Autodesk Inventor part; units mm, degrees
ref_plane "YZ Plane" through (0, 0, 0) normal (1, 0, 0) x (0, 1, 0)
ref_plane "XZ Plane" through (0, 0, 0) normal (0, 1, 0) x (-1, 0, 0)
ref_plane "XY Plane" through (0, 0, 0) normal (0, 0, 1) x (1, 0, 0)
sketch "Skizze1" plane through (0, 0, 0) normal (0, 0, 1) x (1, 0, 0)
  line L0 (-68.016, 1.808) -> (67.584, 1.808)
  line L1 (67.584, 1.808) -> (67.584, -2.192)
  line L2 (67.584, -2.192) -> (-68.016, -2.192)
  line L3 (-68.016, -2.192) -> (-68.016, 1.808)
  line L4 (-68.016, 1.808) -> (67.584, -2.192) construction
  line L5 (67.584, 1.808) -> (-68.016, -2.192) construction
  point P0 (0, 0)
  point P1 (-0.216, -0.192)
  point P2 (-0.216, -0.192)
  dimension "d0" = 135.6
  dimension "d1" = 4
extrude "Extrusion1" add sketch "Skizze1" along normal mid plane 3.25
ref_plane "Arbeitsebene1" through (-68.016, -0.192, 1.625) normal (0, -1, 0) x (1, 0, 0)
sketch "Skizze2" plane through (-68.016, -0.192, 1.625) normal (0, -1, 0) x (1, 0, 0)
  line L0 (0, -3.25) -> (0, 0)
  line L1 (0, -3.25) -> (135.6, -3.25)
  line L2 (0, 0) -> (2.85, 0)
  line L3 (2.85, 0) -> (2.85, -3.25)
  line L4 (2.85, -3.25) -> (0, -3.25)
  line L5 (0, -3.25) -> (0, 0)
  line L6 (0, 0) -> (0, 1.75)
  line L7 (0, 1.75) -> (2.85, 0)
  line L8 (135.6, -3.25) -> (135.6, 0)
  line L9 (135.6, 0) -> (132.75, 0)
  line L10 (132.75, 0) -> (132.75, -3.25)
  line L11 (132.75, -3.25) -> (135.6, -3.25)
  line L12 (135.6, -3.25) -> (135.6, 0)
  line L13 (135.6, 0) -> (135.6, 1.75)
  line L14 (135.6, 1.75) -> (132.75, 0)
  point P0 (68.016, -1.625)
  dimension "d4" = 2.85
  dimension "d5" = 1.75
  dimension "d6" = 2.85
extrude "Extrusion2" add sketch "Skizze2" along normal mid plane 19.7
sketch "Skizze3" plane through (0, 0, 1.625) normal (0, 0, 1) x (1, 0, 0)
  circle A0 centre (0, 0) radius 9.95
  dimension "d9" = 19.9
extrude "Extrusion3" cut sketch "Skizze3" against normal through all
sketch "Skizze4" plane through (0, 0, -1.625) normal (0, 0, -1) x (-1, 0, 0)
  line L0 (0.0981, 0.0423) -> (6.2481, 0.0423) construction
  circle A0 centre (0.0003, -0.1906) radius 7.9
  circle A1 centre (0.0003, -0.1906) radius 10.7
  line L1 (-24.5997, -4.0906) -> (24.6003, -4.0906)
  point P0 (-11.2287, 0.0116)
  point P1 (11.2713, 0.0116)
  point P2 (0.0213, -0.1938)
  point P3 (6.8705, -4.0906)
  point P4 (9.9642, -4.0906)
  point P5 (-9.9636, -4.0906)
  point P6 (-6.8699, -4.0906)
  dimension "d27" = 2.8
  dimension "d28" = 15.8
  dimension "d29" = 3.9
extrude "Extrusion4" add sketch "Skizze4" against normal blind 7 contours A0 L1 A1 picked at (9.6695, 0.6375)
sketch "Skizze5" plane through (0, 0, 1.625) normal (0, 0, 1) x (1, 0, 0)
  line L0 (-10.512, 1.808) -> (-65.166, 1.808)
  line L1 (-10.5115, -2.192) -> (-65.166, -2.192)
  line L2 (-10.2094, 1.808) -> (-63.2094, 1.808)
  line L3 (-63.2094, 1.808) -> (-63.2094, -2.192)
  line L4 (-63.2094, -2.192) -> (-10.2094, -2.192)
  line L5 (-10.2094, -2.192) -> (-10.2094, 1.808)
  line L6 (10.5109, -2.192) -> (64.734, -2.192)
  line L7 (9.6345, 1.808) -> (62.6345, 1.808)
  line L8 (62.6345, 1.808) -> (62.6345, -2.192)
  line L9 (62.6345, -2.192) -> (9.6345, -2.192)
  line L10 (9.6345, -2.192) -> (9.6345, 1.808)
  point P0 (0, 0)
  point P1 (-8.6889, 1.808)
  point P2 (-8.6001, -2.192)
  point P3 (8.6889, 1.808)
  point P4 (8.6001, -2.192)
  point P5 (8.251, -2.192)
  point P6 (-13.2094, -2.192)
  point P7 (-63.2094, 1.808)
  point P8 (62.6345, -2.192)
  point P9 (-7.3561, 1.808)
  point P10 (-7.2509, -2.192)
  point P11 (7.2509, -2.192)
  dimension "d17" = 53
  dimension "d18" = 53
extrude "Extrusion5" add sketch "Skizze5" along normal blind 2.25
sketch "Skizze6" plane through (-65.166, -2.192, -1.625) normal (0, -1, 0) x (1, 0, 0)
  line L0 (1.9566, 5.5) -> (54.6545, 5.5)
  line L1 (1.9566, 5.5) -> (56.9566, 5.5)
  line L2 (56.9566, 5.5) -> (56.9566, 3.25)
  line L3 (56.9566, 3.25) -> (1.9566, 3.25)
  line L4 (1.9566, 3.25) -> (1.9566, 5.5)
  line L5 (56.9566, 5.5) -> (1.9566, 3.25)
  line L6 (127.8005, 3.25) -> (127.8005, 5.5)
  line L7 (127.8005, 5.5) -> (72.8005, 5.5)
  line L8 (72.8005, 5.5) -> (72.8005, 3.25)
  line L9 (72.8005, 3.25) -> (127.8005, 3.25)
  line L10 (127.8005, 3.25) -> (127.8005, 5.5)
  line L11 (72.8005, 5.5) -> (127.8005, 3.25)
  point P0 (65.166, 1.625)
  point P1 (56.5659, 5.5)
  point P2 (54.0951, 5.5)
  point P3 (56.5659, 5.5)
  point P4 (54.0951, 5.5)
  dimension "d21" = 55
  dimension "d22" = 2.25
  dimension "d23" = 55
  dimension "d26" = 2.25
extrude "Extrusion6" cut sketch "Skizze6" against normal through all contours L0 L1 L5 L4 | L11 L7 L6
draft "Flächenverjüngung2" angle 5.7 pull direction (0, 0, -1) faces at (7.1819, -3.4809, 2.5416) fixed edges at (7.642, -2.192, 3.8748) (7.8997, -0.176, 3.875)
properties part number "2024_08_28_Holder_NS14"
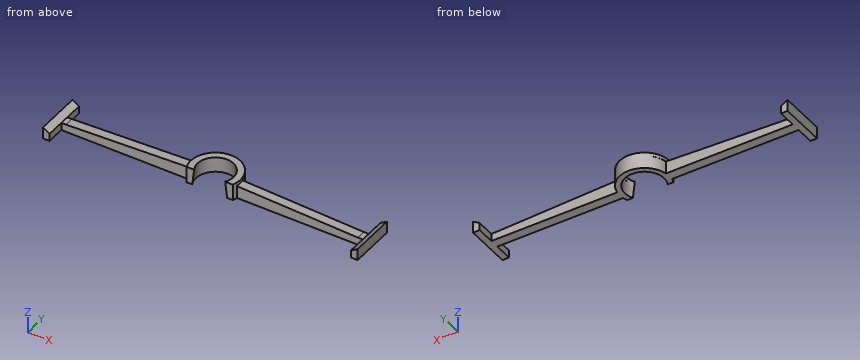
Geometry check sheet. Reference: the model listing, model coordinates, mm. Coordinates: 2 decimals unless noted, no trailing zeros. Order: outer loops, then holes, each group sorted by start corner. A loop starts at its lowest first (then second) coordinate and runs counter-clockwise, first axis right, second up. Notation, with made-up numbers: (50, 27) -> (91, 27) arc R18 ccw to (91, 48) -> close; hole circle Ø1 at (17.25, 72). An arc over 180 degrees is marked (long way). Use a Markdown table: item, result. Add a question column.
1. Cross-section at A-A (y = -6). Enter the section's corners in (x, z) (3 decimals).
2. Material ranges on L1, parallel to X at y = -6.75, z = -1; L2, parallel to X at y = 3, z = -0.75; L3, parallel to Y at x = 34, z = 0.75, recorded low to high.
3. Cross-section at C-C (x = -29). Enter the section's corners in (y, z) (3 decimals), and give its area (3 significant figures).
4. Cross-section at D-D (y = -1). Give the number of separate pieces and of enclosed holes in the cut face, and give its area (3 significant figures).
5. Cross-section at B-B (z = 0.5). Enter the section's corners in (x, y), and give its area (3 significant figures).
6. Go/stop test with flat-tipped pins: pin 1 Ø1.6 at (x, z) = (34.5, 0) entering from -Y; pin 2 Ø0.9 at (x, z) = (-66.5, 1) entering from +Y; pin 3 Ø12 at (x, y) = (-22.5, 0) entering from +Z. Record where each tip stops, or that it passes through.
Filled sheet:
| question | item | result |
|---|---|---|
| 1 | outline | (-68.016, -1.625) -> (-65.166, -1.625) -> (-65.166, 1.625) -> (-68.016, 3.375) -> close; (64.734, -1.625) -> (67.584, -1.625) -> (67.584, 3.375) -> (64.734, 1.625) -> close |
| 2 | L1 | -68.02 to -65.17, 64.73 to 67.58 |
| 2 | L2 | -68.02 to -65.17, -10.21 to -7.73, 7.73 to 10.21, 64.73 to 67.58 |
| 2 | L3 | -2.19 to 1.81 |
| 3 | outline | (-2.192, -1.625) -> (1.808, -1.625) -> (1.808, 3.024) -> (-2.192, 3.024) -> close |
| 3 | area | 18.6 mm2 |
| 4 | separate pieces | 3 |
| 4 | enclosed holes | 0 |
| 4 | area | 524 mm2 |
| 5 | outline | (-68.02, -10.04) -> (-65.17, -10.04) -> (-65.17, -2.19) -> (-10.51, -2.19) arc R10.7 ccw to (-9.96, -4.09) -> (-7.26, -4.09) arc R8.24 cw (long way) to (7.25, -4.09) -> (9.96, -4.09) arc R10.7 ccw to (10.51, -2.19) -> (64.73, -2.19) -> (64.73, -10.04) -> (67.58, -10.04) -> (67.58, 9.66) -> (64.73, 9.66) -> (64.73, 1.81) -> (10.51, 1.81) arc R10.7 ccw to (-10.51, 1.81) -> (-65.17, 1.81) -> (-65.17, 9.66) -> (-68.02, 9.66) -> close |
| 5 | area | 640 mm2 |
| 6 | pin 1 | y = -2.19 |
| 6 | pin 2 | y = 9.66 |
| 6 | pin 3 | z = 3.54 |
